from build123d import *

# Parameters (mm, degrees)
F1_W     = 182.88
F1_H     = 274.32
F2_DEPTH = 121.92
F3_R     = 5.159375
F4_DEPTH = 121.92
F5_W     = 60.96
F5_H     = 152.4
F6_DEPTH = 121.92
F7_R     = 0.79375


with BuildPart() as f2:
    # F1 (on Front) → F2 (new body)
    with BuildSketch(Plane.XZ):
        Rectangle(F1_W, F1_H)
    extrude(amount=-F2_DEPTH)

    # F3 (on face) → F4 (cut)
    with BuildSketch(Plane.XZ):
        with Locations((-60.96, 106.68)):
            Circle(F3_R)
        with Locations((60.96, 106.68)):
            Circle(F3_R)
        with Locations((-60.96, -106.68)):
            Circle(F3_R)
        with Locations((60.96, -106.68)):
            Circle(F3_R)
    extrude(amount=-F4_DEPTH, mode=Mode.SUBTRACT)

    # F5 (on face) → F6 (cut)
    with BuildSketch(Plane.XZ):
        Rectangle(F5_W, F5_H)
    extrude(amount=-F6_DEPTH, mode=Mode.SUBTRACT)

    # F7
    f7_edges = [f2.edges().sort_by_distance(p)[0] for p in [
        (-30.48, 60.96, 76.2),
        (30.48, 60.96, 76.2),
        (30.48, 60.96, -76.2),
        (-30.48, 60.96, -76.2),
    ]]
    fillet(f7_edges, radius=F7_R)


solid = f2.part
Source: CAD feature listing. Evaluate the final solid. Frame: model axes, mm. A direction names the side the tool comes from. Give positions to 0.01 mm unless a question says otherwise; leave off trailing zeros. Write each loop counter-clockwise with the first axis right and the second up, starting at its lowest first coordinate (ties: lowest second). Pieces come first, ordered by that corner, then holes. Notation, with made-up numbers: M 51.25,8 L 83.25,8 A29 ccw 83.25,32 Z; hole C 43.5,36.5 d6. An arc over 180 degrees is marked long. Return JSON: item names as keys, results as strings. Group by question number.
1) Set-up query: faces 4 (the face through (91.44, 60, -2)), 5 (the face through (0, 60, 76.2)). Return all of +Z, -Z, +X, -X, +Y, -Y with unobstructed straight access to the full face (end or side cutting, diameter ignored); none if empty.
2) Pin query (flat end, axial travel): P1, Ø8.5, axis at x = 60.96, z = -106.68, coming from the +Y side. Return the tip coordinate at first contact, or that it passes through.
3) Cut plane A-A, the plane z = -106.68. Output: boundary loops of the cut face in (x, y).
4) Pull-direction query (X, two-part tool) for faces 1 (the face through (-91.44, 60, -2)), 2 (the face through (39, 0, 2)), 3 (the face through (-64.76, 60.11, -103.19)); classes: pulls with the +X half, pulls with the -X half, needs draft (parallel to the pull), parting line crosses it, or undercut.
5) Cut plane B-B, the plane x = 23.5. Output: boundary loops of the cut face in (y, z), plus the area to 3 significant figures.
6) Cut plane D-D, the plane y = 113. Output: boundary loops of the cut face in (x, z), plus the area to 3 significant figures.
7) Material intervals for line 1 along X through (y, z) = (79, -106); line 2 along Z through (x, y) = (-12, 33); line 3 along X through (y, z) = (107.5, 110), sorted ascending. Write a range as [from, to].
8) Cut plane C-C, the plane z = 61.5. Output: boundary loops of the cut face in (x, y).
Recorded:
{
 "1": {"face 4": "+Z, -Z, +X, +Y, -Y", "face 5": "+Y, -Y"},
 "2": {"P1": "passes through"},
 "3": {"outline": "M -91.44,0 L -66.12,0 L -66.12,121.92 L -91.44,121.92 Z; M -55.8,0 L 55.8,0 L 55.8,121.92 L -55.8,121.92 Z; M 66.12,0 L 91.44,0 L 91.44,121.92 L 66.12,121.92 Z"},
 "4": {"face 1": "pulls with the -X half", "face 2": "needs draft", "face 3": "undercut"},
 "5": {"outline": "M 0,-137.16 L 121.92,-137.16 L 121.92,-76.2 L 0,-76.2 Z; M 0,76.2 L 121.92,76.2 L 121.92,137.16 L 0,137.16 Z", "area": "14,900 mm²"},
 "6": {"outline": "M -91.44,-137.16 L 91.44,-137.16 L 91.44,137.16 L -91.44,137.16 Z; hole C -60.96,-106.68 d10.32; hole C -60.96,106.68 d10.32; hole M -30.48,-75.41 A0.79 ccw -29.69,-76.2 L 29.69,-76.2 A0.79 ccw 30.48,-75.41 L 30.48,75.41 A0.79 ccw 29.69,76.2 L -29.69,76.2 A0.79 ccw -30.48,75.41 Z; hole C 60.96,-106.68 d10.32; hole C 60.96,106.68 d10.32", "area": "40,500 mm²"},
 "7": {"line 1": "x = [-91.44, -66.07], [-55.85, 55.85], [66.07, 91.44]", "line 2": "z = [-137.16, -76.2], [76.2, 137.16]", "line 3": "x = [-91.44, -64.91], [-57.01, 57.01], [64.91, 91.44]"},
 "8": {"outline": "M -91.44,0 L -30.48,0 L -30.48,121.92 L -91.44,121.92 Z; M 30.48,0 L 91.44,0 L 91.44,121.92 L 30.48,121.92 Z"}
}
